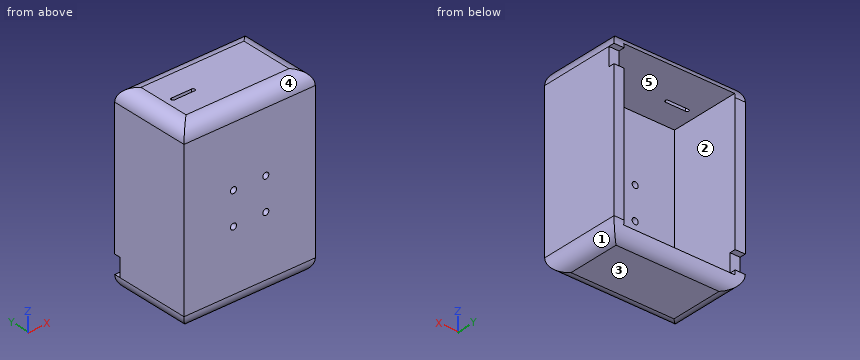
from build123d import *

# Parameters (mm, degrees)
ESBO_O3_W                = 65
ESBO_O3_H                = 90
RESSALTO_EXTRUS_O2_DEPTH = 40
CASCA2_T                 = -5
ESBO_O4_R                = 1.5
CORTE_EXTRUS_O1_DEPTH    = 40
FILETE2_R                = 7
ESBO_O5_W                = 5
ESBO_O5_H                = 9
CORTE_EXTRUS_O2_DEPTH    = 3
ESBO_O7_W                = 5
ESBO_O7_H                = 9
CORTE_EXTRUS_O3_DEPTH    = 3
CORTE_EXTRUS_O4_REACH    = 105.712


with BuildPart() as part:
    # Esboço3 → Ressalto-extrusão2 (new body)
    with BuildSketch(Plane(origin=(0, 0, 0), x_dir=(1, 0, 0), z_dir=(0, 1, 0))):
        Rectangle(ESBO_O3_W, ESBO_O3_H)
    extrude(amount=RESSALTO_EXTRUS_O2_DEPTH)

    # Casca2
    casca2_openings = [part.faces().sort_by_distance(p)[0] for p in [
        (0, 40, 0),
    ]]
    offset(amount=CASCA2_T, openings=casca2_openings, kind=Kind.INTERSECTION)

    # Esboço4 → Corte-extrusão1 (cut)
    with BuildSketch(Plane(origin=(0, 5, 0), x_dir=(1, 0, 0), z_dir=(0, 1, 0))):
        with Locations(Location((-8, 8, 0), (0, 0, 270))):
            Circle(ESBO_O4_R)
        with Locations(Location((8, 8, 0), (0, 0, 90))):
            Circle(ESBO_O4_R)
        with Locations(Location((8, -8, 0), (0, 0, 270))):
            Circle(ESBO_O4_R)
        with Locations(Location((-8, -8, 0), (0, 0, 90))):
            Circle(ESBO_O4_R)
    extrude(amount=-CORTE_EXTRUS_O1_DEPTH, mode=Mode.SUBTRACT)

    # Filete2
    # the kernel refuses this fillet: 7 mm, written as the material it takes off along each edge
    with BuildSketch(Plane(origin=(32.5, -17.5, -45), x_dir=(0, 0, 1), z_dir=(0, 1, 0)), Plane(origin=(32.5, -17.5, 45), x_dir=(-1, 0, 0), z_dir=(0, 1, 0))) as filete2_piece_1:
        with BuildLine():
            CenterArc((FILETE2_R, -FILETE2_R), FILETE2_R, 90, 90)
            Line((0, -FILETE2_R), (0, 0))
            Line((0, 0), (FILETE2_R, 0))
        make_face()
    extrude(amount=75, mode=Mode.SUBTRACT)
    with BuildSketch(Plane(origin=(50, 40, -45), x_dir=(0, 0, 1), z_dir=(-1, 0, 0)), Plane(origin=(-50, 0, 45), x_dir=(0, 1, 0), z_dir=(1, 0, 0))) as filete2_piece_2:
        with BuildLine():
            CenterArc((FILETE2_R, -FILETE2_R), FILETE2_R, 90, 90)
            Line((0, -FILETE2_R), (0, 0))
            Line((0, 0), (FILETE2_R, 0))
        make_face()
    extrude(amount=100, mode=Mode.SUBTRACT)
    with BuildSketch(Plane(origin=(-32.5, -17.5, -45), x_dir=(0, 0, 1), z_dir=(0, 1, 0)), Plane(origin=(-32.5, -17.5, 45), x_dir=(1, 0, 0), z_dir=(0, 1, 0))) as filete2_piece_3:
        with BuildLine():
            CenterArc((FILETE2_R, FILETE2_R), FILETE2_R, 180, 90)
            Line((0, FILETE2_R), (0, 0))
            Line((0, 0), (FILETE2_R, 0))
        make_face()
    extrude(amount=75, mode=Mode.SUBTRACT)
    with BuildSketch(Plane(origin=(50, 0, -45), x_dir=(0, 0, 1), z_dir=(-1, 0, 0)), Plane(origin=(-50, 40, 45), x_dir=(0, -1, 0), z_dir=(1, 0, 0))) as filete2_piece_4:
        with BuildLine():
            CenterArc((FILETE2_R, FILETE2_R), FILETE2_R, 180, 90)
            Line((0, FILETE2_R), (0, 0))
            Line((0, 0), (FILETE2_R, 0))
        make_face()
    extrude(amount=100, mode=Mode.SUBTRACT)

    # Esboço5 → Corte-extrusão2 (cut)
    with BuildSketch(Plane(origin=(0, 40, 0), x_dir=(1, 0, 0), z_dir=(0, 1, 0))):
        with Locations((-30, 33.5)):
            Rectangle(ESBO_O5_W, ESBO_O5_H)
    extrude(amount=-CORTE_EXTRUS_O2_DEPTH, mode=Mode.SUBTRACT)

    # Esboço7 → Corte-extrusão3 (cut)
    with BuildSketch(Plane(origin=(0, 40, 0), x_dir=(1, 0, 0), z_dir=(0, 1, 0))):
        with Locations((30, -33.5)):
            Rectangle(ESBO_O7_W, ESBO_O7_H)
    extrude(amount=-CORTE_EXTRUS_O3_DEPTH, mode=Mode.SUBTRACT)

    # Esboço8 → Corte-extrusão4 (cut, up to next)
    with BuildSketch(Plane.XY.offset(45), mode=Mode.PRIVATE) as corte_extrus_o4_sk1:
        with BuildLine():
            Line((-21.8264162, 19.698053531), (-11.8264162, 19.698053531))
            ThreePointArc((-11.8264162, 19.698053531), (-10.963712002, 18.835349333), (-11.8264162, 17.972645136))
            Line((-11.8264162, 17.972645136), (-21.8264162, 17.972645136))
            ThreePointArc((-21.8264162, 17.972645136), (-22.689120398, 18.835349333), (-21.8264162, 19.698053531))
        make_face()
    corte_extrus_o4_tool1 = extrude(corte_extrus_o4_sk1.sketch, amount=-CORTE_EXTRUS_O4_REACH, mode=Mode.PRIVATE) & part.part
    add(corte_extrus_o4_tool1.solids().sort_by_distance((-16.826416, 18.835349, 45))[0], mode=Mode.SUBTRACT)


solid = part.part
Source: CAD feature listing. Evaluate the final solid. Frame: model axes, mm. Face numbers are marked on the shaded views. A direction names the side the tool comes from. Round coordinates to 2 decimals unless told otherwise and drop trailing zeros. Loops run counter-clockwise (first coordinate to the right, second up) from the corner with the lowest first, then second, coordinate; pieces in that order, holes last.
Q1. Ray query, line 1 (X direction, y = 3.35, z = 8); line 2 (Z direction, x = -0.5, y = 12); line 3 (X direction, y = 21.5, z = 6). Return the intervals inside material, ascending.
Q2. Section A-A, the plane z = 8. Return loops of the section in (x, y).
Q3. First-contact query: P1, Ø2.5, axis at x = -8, z = 8, coming from the +Y side; P2, Ø5, axis at x = -8, z = -8, coming from the -Y side; P3, Ø4, axis at x = -1, z = 25.5, coming from the +Y side; P4, Ø1.5, axis at x = 30, z = 31.5, coming from the +Y side. Flat tips, straight axial feed; report the tip coordinate or a pass-through.
Q4. Section C-C, the plane x = -8. Return loops of the section in (y, z), plus the area to 3 significant figures.
Q5. Section D-D, the plane z = -31. Return loops of the section in (x, y), plus the area to 3 significant figures.
Q6. Mould query, pull axis Z, two halves, no side actions, for the marked faces 3, 4 and 5. Classes: pulls with the +Z half, pulls with the -Z half, needs draft (parallel to the pull), parting line crosses it, or undercut.
Q7. Section B-B, the plane y = 10. Return loops of the section in (x, z), plus the area to 3 significant figures.
Q8. Access query for the marked faces 1 and 2. Directions: +Z, -Z, +X, -X, +Y, -Y. A direction counts if a zero-diameter tool reaches every point of the face in a straight line with its end or side. Return the directions, or none.
Solutions:
1. line 1: x = -32.5 to -9.5, -6.5 to 6.5, 9.5 to 32.5
1. line 2: z = -45 to -40, 40 to 45
1. line 3: x = -32.5 to -27.5, 27.5 to 32.5
2. outline: (-32.5, 0) - (-9.5, 0) - (-9.5, 5) - (-27.5, 5) - (-27.5, 40) - (-32.5, 40) - close; (-6.5, 0) - (6.5, 0) - (6.5, 5) - (-6.5, 5) - close; (9.5, 0) - (32.5, 0) - (32.5, 40) - (27.5, 40) - (27.5, 5) - (9.5, 5) - close
3. P1: passes through
3. P2: stops at y = 0
3. P3: stops at y = 5
3. P4: stops at y = 37
4. outline: (0, -38) arc R7 ccw to (7, -45) - (33, -45) arc R7 ccw to (39.71, -40) - (5, -40) - (5, -9.5) - (0, -9.5) - close; (0, -6.5) - (5, -6.5) - (5, 6.5) - (0, 6.5) - close; (0, 9.5) - (5, 9.5) - (5, 40) - (39.71, 40) arc R7 ccw to (33, 45) - (7, 45) arc R7 ccw to (0, 38) - close
4. area: 728 mm2
5. outline: (-32.5, 0) - (32.5, 0) - (32.5, 40) - (27.5, 40) - (27.5, 5) - (-27.5, 5) - (-27.5, 37) - (-32.5, 37) - close
5. area: 660 mm2
6. face 3: pulls with the -Z half
6. face 4: pulls with the +Z half
6. face 5: undercut
7. outline: (-32.5, -38) arc R7 ccw to (-25.5, -45) - (25.5, -45) arc R7 ccw to (32.5, -38) - (32.5, 38) arc R7 ccw to (25.5, 45) - (-25.5, 45) arc R7 ccw to (-32.5, 38) - close; hole (-27.5, -40) - (27.5, -40) - (27.5, 40) - (-27.5, 40) - close
7. area: 1,410 mm2
8. face 1: -Z, +X, +Y, -Y
8. face 2: +Y
